Geometry check sheet. Reference: drawing and pictorial views, mm from the part's lowest x, y, z. Coordinates: 2 decimals unless noted, no trailing zeros. Loops run counter-clockwise (first coordinate to the right, second up) from the corner with the lowest first, then second, coordinate; pieces in that order, holes last. Notation, with made-up numbers: (55.25, 35) - (59.25, 35) arc R12 ccw to (59.25, 55) - close; hole circle Ø7 at (19, 43.5). An arc over 180 degrees is marked (long way). One line per item, written item: value.
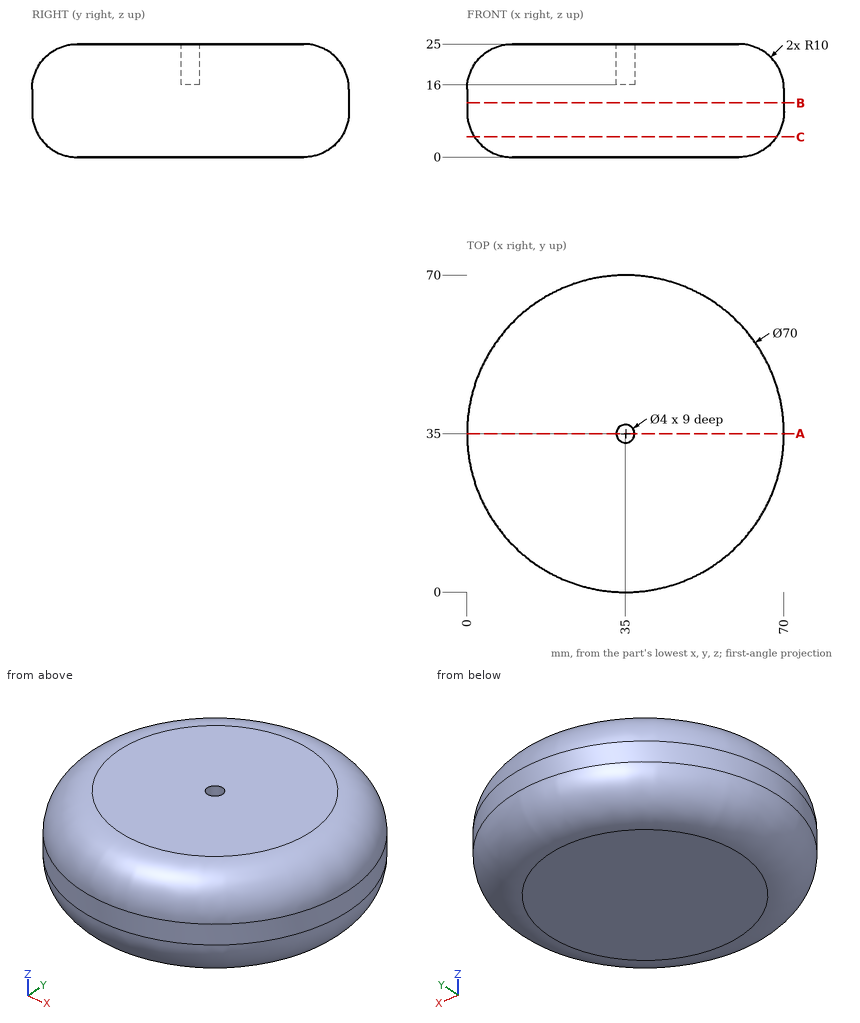
(1) Material ranges on probe 1 along Y at (x, z) = (35, 20.5); probe 2 along Y at (x, z) = (35, 20.75); probe 3 along X at (y, z) = (47, 16), recorded low to high. Write a range as from..to.
Reply:
probe 1: 1.65..33, 37..68.35
probe 2: 1.82..33, 37..68.18
probe 3: 2.17..67.83
(2) Go/stop test with flat-tipped pins: pin 1 Ø5 at (x, z) = (22, 6) entering from +Y; pin 2 Ø2 at (x, z) = (19, 19) entering from +Y; pin 3 Ø3 at (y, z) = (14, 6.5) entering from +X. Record where each tip stops, or that it passes through.
Reply:
pin 1: y = 67.89
pin 2: y = 65.86
pin 3: x = 63.46
(3) Cross-section at C-C on z = 4.5. Record the cut outline in (x, y), and give its area (3 significant figures).
Reply:
outline: circle Ø66.7 at (35, 35)
area: 3,490 mm2
(4) Cross-section at A-A on y = 35. Record the cut outline in (x, z).
Reply:
outline: (0, 10) arc R10 ccw to (10, 0) - (60, 0) arc R10 ccw to (70, 10) - (70, 15) arc R10 ccw to (60, 25) - (37, 25) - (37, 16) - (33, 16) - (33, 25) - (10, 25) arc R10 ccw to (0, 15) - close
(5) Cross-section at B-B on z = 12. Record the cut outline in (x, y).
Reply:
outline: circle Ø70 at (35, 35)
